```python
from build123d import *

# Parameters (mm, degrees)
CUT_EXTRUDE_1_DEPTH = 0.4
CHAMFER_1_SIZE      = 0.2


with BuildPart() as part:
    # 草图1 → 旋转1 (revolve)
    with BuildSketch(Plane.XY, mode=Mode.PRIVATE) as revolve_1_sk:
        Polygon((0, 0), (0, -2.4), (0.2, -2.4), (2.3, -1.25), (14, -1.25), (14, 0), align=None)
    revolve(revolve_1_sk.sketch.rotate(Axis((14, 0, 0), (-1, 0, 0)), 180), axis=Axis((14, 0, 0), (-1, 0, 0)))

    # 草图2 → 切除-拉伸1 (cut)
    with BuildSketch(Plane.ZY):
        Polygon((0.866025404, 0), (0.433012702, 0.75), (-0.433012702, 0.75), (-0.866025404, 0), (-0.433012702, -0.75), (0.433012702, -0.75), align=None)
    extrude(amount=-CUT_EXTRUDE_1_DEPTH, mode=Mode.SUBTRACT)

    # 倒角1
    chamfer_1_edges = [part.edges().sort_by_distance(p)[0] for p in [
        (14, -1.25, 0),
    ]]
    chamfer(chamfer_1_edges, length=CHAMFER_1_SIZE)


solid = part.part
```
CAD build for the part. Positions are in the model's coordinates, mm. Round coordinates to 2 decimals unless told otherwise and drop trailing zeros. Order: outer loops, then holes, each group sorted by start corner. A loop starts at its lowest first (then second) coordinate and runs counter-clockwise, first axis right, second up.
Item 1: Probe line 1 along Y through (x, z) = (12.25, -0.05); line 2 along Z through (x, y) = (7, 1.05); line 3 along Y through (x, z) = (12, 0.9). List the from-to ranges inside material, lowest first.
Item 2: Mould opens along Y. For faces 1 (the face through (0.4, 0, 0)), 2 (the face through (8.13, -1.25, -0.05)), 3 (the face through (0, 1, -1)) say: pulls with the +Y half, pulls with the -Y half, needs draft (parallel to the pull), parting line crosses it, or undercut.
Item 3: Saw through at B-B on x = 6.75. Write the cut outline in (y, z).
Item 4: Pin check, flat tips, straight feed: pin 1 (1 mm diameter, centred on x = 5.5, z = 1, fed in from +Y); pin 2 (1 mm diameter, centred on x = 7, z = -2, fed in from -Y); pin 3 (0.8 mm diameter, centred on y = 0, z = 0, fed in from -X). Stop position of each tip, or through.
Item 5: Saw through at A-A on z = 0. Write the cut outline in (x, y).
Reported:
1. line 1: y = -1.25 to 1.25
1. line 2: z = -0.68 to 0.68
1. line 3: y = -0.87 to 0.87
2. face 1: undercut
2. face 2: parting line crosses it
2. face 3: needs draft
3. outline: circle Ø2.5 at (0, 0)
4. pin 1: stops at y = 1.15
4. pin 2: passes through
4. pin 3: stops at x = 0.4
5. outline: (0, -2.4) - (0.2, -2.4) - (2.3, -1.25) - (13.8, -1.25) - (14, -1.05) - (14, 1.05) - (13.8, 1.25) - (2.3, 1.25) - (0.2, 2.4) - (0, 2.4) - (0, 0.75) - (0.4, 0.75) - (0.4, -0.75) - (0, -0.75) - close
